Design review of the part built by this model. Coordinates are the model's own, in mm. Face numbers are marked on the shaded views. A direction names the side the tool comes from. Coordinates: 2 decimals unless noted, no trailing zeros. Loops run counter-clockwise (first coordinate to the right, second up) from the corner with the lowest first, then second, coordinate; pieces in that order, holes last. Notation, with made-up numbers: (21.25, 0) -> (35.25, 0) arc R28 ccw to (35.25, 32) -> close; hole circle Ø6 at (5.25, -29). An arc over 180 degrees is marked (long way). Answer in a Markdown table with one row per item.
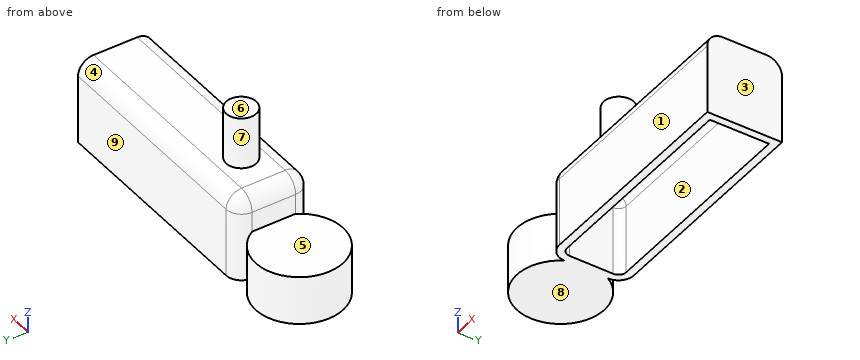
```python
from build123d import *

# Parameters (mm, degrees)
F1_DEPTH = 27.686
F2_R     = 5.08
F3_T     = -2.54
F4_R     = 4.9426127615
F5_DEPTH = 17.018
F7_DEPTH = 16.002


with BuildPart() as f1:
    # F0 (on Top) → F1 (new body)
    with BuildSketch(Plane.XY):
        Polygon((-77.3243010044, 0), (0, 0), (0, 24.5208609849), (-77.4464830756, 24.5208609849), align=None)
    extrude(amount=F1_DEPTH)

    # F2
    f2_edges = [f1.edges().sort_by_distance(p)[0] for p in [
        (-77.446483, 24.520861, 13.843),
        (-38.723242, 24.520861, 27.686),
        (-77.385392, 12.26043, 27.686),
        (-38.662151, 0, 27.686),
        (-77.324301, 0, 13.843),
    ]]
    fillet(f2_edges, radius=F2_R)

    # F3
    f3_openings = [f1.faces().sort_by_distance(p)[0] for p in [
        (-38.472172, 12.262955, 0),
    ]]
    offset(amount=F3_T, openings=f3_openings)

    # F4 (on face) → F5 (join)
    with BuildSketch(Plane.XY.offset(27.686)):
        with Locations((-60.7563629746, 11.7522832006)):
            Circle(F4_R)
    extrude(amount=F5_DEPTH)

    # F6 (on face) → F7 (join)
    with BuildSketch(Plane(origin=(0, 0, 0), x_dir=(1, 0, 0), z_dir=(0, 0, -1))):
        with BuildLine():
            Line((-77.4210444248, -19.4155487735), (-77.3494874048, -5.0546877886))
            ThreePointArc((-77.3494874048, -5.0546877886), (-104.1229765697, -12.1018901343), (-77.4210444248, -19.4155487735))
        make_face()
    extrude(amount=-F7_DEPTH)


solid = f1.part
```
(1) To check wall thickness, follow probe 1 along Y at (x, z) = (-56.5, 7); probe 2 along X at (y, z) = (3, 3); probe 3 along Z at (x, y) = (-64, 6.75). State the ranges of each line that lie inside material, in increasing order.
Evaluation:
| item | result |
|---|---|
| probe 1 | y = 0 to 2.54, 21.98 to 24.52 |
| probe 2 | x = -100.8 to -78.78, -76.9 to -73.73, -2.54 to 0 |
| probe 3 | z = 25.15 to 27.69 |
(2) Tool access review of the marked faces 5, 6, 7, 8 and 9: name each direction out of +Z, -Z, +X, -X, +Y, -Y from which nothing blocks a thin tool from reaching the whole face with its end or side.
Evaluation:
| item | result |
|---|---|
| face 5 | +Z, -X, +Y, -Y |
| face 6 | +Z, +X, -X, +Y, -Y |
| face 7 | +Z |
| face 8 | -Z, +X, -X, +Y, -Y |
| face 9 | +Z, -Z, +X, +Y |
(3) Draft analysis for pull direction Y (two halves, no side actions). For the marked faces 1, 2, 3 and 4, state which applies: pulls with the +Y half, pulls with the -Y half, needs draft (parallel to the pull), parting line crosses it, or undercut.
Evaluation:
| item | result |
|---|---|
| face 1 | pulls with the -Y half |
| face 2 | undercut |
| face 3 | needs draft |
| face 4 | pulls with the +Y half |
(4) Take a section at D-D on x = -58. Give the boundary of the cut face in (y, z).
Evaluation:
| item | result |
|---|---|
| outline | (0, 0) -> (2.54, 0) -> (2.54, 22.61) arc R2.54 cw to (5.08, 25.15) -> (19.44, 25.15) arc R2.54 cw to (21.98, 22.61) -> (21.98, 0) -> (24.52, 0) -> (24.52, 22.61) arc R5.08 ccw to (19.44, 27.69) -> (15.85, 27.69) -> (15.85, 44.7) -> (7.65, 44.7) -> (7.65, 27.69) -> (5.08, 27.69) arc R5.08 ccw to (0, 22.61) -> close |
(5) Take a section at B-B on x = -21. Give the boundary of the cut face in (y, z).
Evaluation:
| item | result |
|---|---|
| outline | (0, 0) -> (2.54, 0) -> (2.54, 22.61) arc R2.54 cw to (5.08, 25.15) -> (19.44, 25.15) arc R2.54 cw to (21.98, 22.61) -> (21.98, 0) -> (24.52, 0) -> (24.52, 22.61) arc R5.08 ccw to (19.44, 27.69) -> (5.08, 27.69) arc R5.08 ccw to (0, 22.61) -> close |
(6) Take a section at C-C on z = 20. Give the boundary of the cut face in (x, y), and give its area (3 significant figures).
Evaluation:
| item | result |
|---|---|
| outline | (-77.42, 19.42) -> (-77.35, 5.05) arc R5.08 ccw to (-72.27, 0) -> (0, 0) -> (0, 24.52) -> (-72.34, 24.52) arc R5.08 ccw to start; hole (-74.88, 19.43) -> (-74.81, 5.07) arc R2.54 ccw to (-72.27, 2.54) -> (-2.54, 2.54) -> (-2.54, 21.98) -> (-72.34, 21.98) arc R2.54 ccw to start |
| area | 484 mm² |
(7) Take a section at A-A on z = 12.5. Give the boundary of the cut face in (x, y), and give its area (3 significant figures).
Evaluation:
| item | result |
|---|---|
| outline | (-77.42, 19.42) arc R14.33 ccw (long way) to (-77.35, 5.05) arc R5.08 ccw to (-72.27, 0) -> (0, 0) -> (0, 24.52) -> (-72.34, 24.52) arc R5.08 ccw to start; hole (-74.88, 19.43) -> (-74.81, 5.07) arc R2.54 ccw to (-72.27, 2.54) -> (-2.54, 2.54) -> (-2.54, 21.98) -> (-72.34, 21.98) arc R2.54 ccw to start |
| area | 1,110 mm² |
(8) For pin 1 (2 mm diameter, centred on x = -75.5, z = 13, fed in from +Y); pin 2 (11.5 mm diameter, centred on x = -33, z = 10.5, fed in from -Y); pin 3 (3 mm diameter, centred on x = -67, z = 16, fed in from +Y); pin 4 (4 mm diameter, centred on x = -56.5, y = 3.5, fed in from -Z), all flat-tipped, find the tip position at first contact; note any pin that passes through.
Evaluation:
| item | result |
|---|---|
| pin 1 | stops at y = 24.04 |
| pin 2 | stops at y = 0 |
| pin 3 | stops at y = 24.52 |
| pin 4 | stops at z = 0 |
